Source: CAD feature listing. Evaluate the final solid. Frame: model axes, mm. A direction names the side the tool comes from. Coordinates: 2 decimals unless noted, no trailing zeros. Loops run counter-clockwise (first coordinate to the right, second up) from the corner with the lowest first, then second, coordinate; pieces in that order, holes last.
Item 1: Section query D-D, the plane x = 15. Return the cut outline in (y, z) (3 decimals).
Item 2: Section query B-B, the plane y = 2.5. Return the cut outline in (x, z) (3 decimals), then the cut area to 3 significant figures.
Item 3: Pull-direction query (Z, two-part tool) for faces 6 (the cylindrical face through (-8.926, -0.986, -41.626)), 7 (the flat face through (10.25, 7, -13)), 8 (the flat face through (0, -2, -53)); classes: +Z half, -Z half, draft (parallel to the pull), parting line (faces both ways), or undercut.
Item 4: Pin query (flat end, axial travel): pin 1 Ø5.5 at (x, z) = (-25.5, 24) entering from +Y; pin 2 Ø1 at (x, y) = (13.5, 9) entering from +Z; pin 3 Ø4 at (x, y) = (-1, 10) entering from -Z. Return the tip coordinate at first contact, or that it passes through.
Item 5: Reachability of faces 1 (the flat face through (-24.509, -1.479, -7.868)), 2 (the cylindrical face through (26.325, -2.535, -44.286)), 3 (the flat face through (-31, -2, -13)), 4 (the flat face through (20.4, 8, -11)), 5 (the flat face through (-14, 4.5, -13)) from +Z, -Z, +X, -X, +Y, -Y: full face, straight path, thin tool, end or side. Return the list, or none.
Item 6: Section query A-A, the plane z = -16. Return the cut outline in (x, y), then the cut area to 3 significant figures.
Item 7: Line query: probe 1 along X at (y, z) = (-3, -21.5); probe 2 along X at (y, z) = (-0.9, 24) (3 decimals); probe 3 along Z at (x, y) = (-21, -1.2). Output: solid intervals per line, ascending.
Item 8: Section query C-C, the plane z = 14. Return the cut outline in (x, y).
```python
from build123d import *

# Parameters (mm, degrees)
F1_W           = 31
F1_H           = 82
F2_DEPTH       = 5
F3_D           = 4.5
F3_CBORE_D     = 6.75
F3_CBORE_DEPTH = 2
F4_DEPTH       = 5
F5_DEPTH       = 2
F6_START       = 0.4
F0_R           = 1.35
F6_DEPTH       = 4.601
F7_D           = 3
F8_R           = 1.5
F9_DEPTH       = 3
F11_DEPTH      = 16.5
F15_D          = 4.25
F16_D          = 3
F18_R          = 2.125
F19_DEPTH      = 5.5
F20_W          = 3
F20_H          = 5
F21_DEPTH      = 3.75
F22_W          = 2.5
F22_H          = 5
F23_DEPTH      = 3.65
F24_R          = 1
F25_DEPTH      = 4
F25_DEPTH_BACK = 5.001
F26_R          = 0.3


# Not quite as in the source:
# - a pattern or mirror of a feature is missing from the dataset's text; its kind, count and spacing are read off the source's solid


with BuildPart() as f2:
    # F1 (on Front) → F2 (new body)
    with BuildSketch(Plane.XZ):
        with Locations((-15.5, -12)):
            Rectangle(F1_W, F1_H)
        with Locations((15.5, -12)):
            Rectangle(F1_W, F1_H)
    extrude(amount=F2_DEPTH)

    # F3 (through all)
    with Locations(Plane(origin=(0, 0, 0), x_dir=(1, 0, 0), z_dir=(0, 1, 0))):
        with Locations((24.75, -24), (6.75, -24), (-6.75, -24), (-24.75, -24), (-24.75, 0), (-6.75, 0), (6.75, 0), (24.75, 0)):
            CounterBoreHole(F3_D / 2, F3_CBORE_D / 2, F3_CBORE_DEPTH)

    # F0 (on Front) → F4 (cut, through all)
    with BuildSketch(Plane.XZ):
        with BuildLine():
            ThreePointArc((6.75, -23), (9, -25.25), (11.25, -23))
            Line((11.25, -23), (11.25, -21))
            ThreePointArc((11.25, -21), (9, -18.75), (6.75, -21))
            Line((6.75, -21), (6.75, -23))
        make_face()
        with BuildLine():
            Line((-6.75, -23), (-6.75, -21))
            ThreePointArc((-6.75, -21), (-9, -18.75), (-11.25, -21))
            Line((-11.25, -21), (-11.25, -23))
            ThreePointArc((-11.25, -23), (-9, -25.25), (-6.75, -23))
        make_face()
        with BuildLine():
            ThreePointArc((6.75, -47), (9, -49.25), (11.25, -47))
            Line((11.25, -47), (11.25, -45))
            ThreePointArc((11.25, -45), (9, -42.75), (6.75, -45))
            Line((6.75, -45), (6.75, -47))
        make_face()
        with BuildLine():
            Line((-6.75, -47), (-6.75, -45))
            ThreePointArc((-6.75, -45), (-9, -42.75), (-11.25, -45))
            Line((-11.25, -45), (-11.25, -47))
            ThreePointArc((-11.25, -47), (-9, -49.25), (-6.75, -47))
        make_face()
    extrude(amount=F4_DEPTH, mode=Mode.SUBTRACT)

    # F0 (on Front) → F5 (cut)
    with BuildSketch(Plane.XZ):
        with BuildLine():
            ThreePointArc((12.375, -21), (9, -17.625), (5.625, -21))
            Line((5.625, -21), (5.625, -23))
            ThreePointArc((5.625, -23), (9, -26.375), (12.375, -23))
            Line((12.375, -23), (12.375, -21))
        make_face()
        with BuildLine():
            Line((11.25, -21), (11.25, -23))
            ThreePointArc((11.25, -23), (9, -25.25), (6.75, -23))
            Line((6.75, -23), (6.75, -21))
            ThreePointArc((6.75, -21), (9, -18.75), (11.25, -21))
        make_face(mode=Mode.SUBTRACT)
        with BuildLine():
            Line((-5.625, -23), (-5.625, -21))
            ThreePointArc((-5.625, -21), (-9, -17.625), (-12.375, -21))
            Line((-12.375, -21), (-12.375, -23))
            ThreePointArc((-12.375, -23), (-9, -26.375), (-5.625, -23))
        make_face()
        with BuildLine():
            ThreePointArc((-11.25, -21), (-9, -18.75), (-6.75, -21))
            Line((-6.75, -21), (-6.75, -23))
            ThreePointArc((-6.75, -23), (-9, -25.25), (-11.25, -23))
            Line((-11.25, -23), (-11.25, -21))
        make_face(mode=Mode.SUBTRACT)
        with BuildLine():
            Line((-5.625, -47), (-5.625, -45))
            ThreePointArc((-5.625, -45), (-9, -41.625), (-12.375, -45))
            Line((-12.375, -45), (-12.375, -47))
            ThreePointArc((-12.375, -47), (-9, -50.375), (-5.625, -47))
        make_face()
        with BuildLine():
            ThreePointArc((-11.25, -45), (-9, -42.75), (-6.75, -45))
            Line((-6.75, -45), (-6.75, -47))
            ThreePointArc((-6.75, -47), (-9, -49.25), (-11.25, -47))
            Line((-11.25, -47), (-11.25, -45))
        make_face(mode=Mode.SUBTRACT)
        with BuildLine():
            ThreePointArc((12.375, -45), (9, -41.625), (5.625, -45))
            Line((5.625, -45), (5.625, -47))
            ThreePointArc((5.625, -47), (9, -50.375), (12.375, -47))
            Line((12.375, -47), (12.375, -45))
        make_face()
        with BuildLine():
            Line((11.25, -45), (11.25, -47))
            ThreePointArc((11.25, -47), (9, -49.25), (6.75, -47))
            Line((6.75, -47), (6.75, -45))
            ThreePointArc((6.75, -45), (9, -42.75), (11.25, -45))
        make_face(mode=Mode.SUBTRACT)
    extrude(amount=F5_DEPTH, mode=Mode.SUBTRACT)

    # F0 (on Front) → F6 (cut)
    with BuildSketch(Plane.XZ.offset(F6_START)):
        with Locations((-19, -21.5)):
            Circle(F0_R)
        with Locations((19, -21.5)):
            Circle(F0_R)
    extrude(amount=F6_DEPTH, mode=Mode.SUBTRACT)

    # F7 (through all)
    with Locations(Plane(origin=(0, 0, 0), x_dir=(1, 0, 0), z_dir=(0, 1, 0))):
        with Locations((26, 10.5), (-26, 10.5)):
            Hole(F7_D / 2)

    # F8 (on face) → F9 (cut)
    with BuildSketch(Plane(origin=(0, 0, 0), x_dir=(-1, 0, 0), z_dir=(0, 1, 0))):
        Polygon((29.025, -12.2464845643), (29.025, -8.7535154357), (26, -7.0070308714), (22.975, -8.7535154357), (22.975, -12.2464845643), (26, -13.9929691286), align=None)
        with Locations((26, -10.5)):
            Circle(F8_R, mode=Mode.SUBTRACT)
        Polygon((-22.975, -12.2464845643), (-22.975, -8.7535154357), (-26, -7.0070308714), (-29.025, -8.7535154357), (-29.025, -12.2464845643), (-26, -13.9929691286), align=None)
        with Locations((-26, -10.5)):
            Circle(F8_R, mode=Mode.SUBTRACT)
    extrude(amount=-F9_DEPTH, mode=Mode.SUBTRACT)

    # F10 (on face) → F11 (join)
    with BuildSketch(Plane(origin=(0, 0, 0), x_dir=(-1, 0, 0), z_dir=(0, 1, 0))):
        Polygon((-7.9, -5), (-20.4, -5), (-20.4, -17.25), (-7.9, -17.25), (-7.9, -14.7), (-5.9, -14.7), (-5.9, -8.7), (-7.9, -8.7), align=None)
        Polygon((0.1, -5), (-7.9, -5), (-7.9, -8.7), (-5.9, -8.7), (-5.9, -14.7), (-7.9, -14.7), (-7.9, -17.25), (0.1, -17.25), (20.6, -17.25), (20.6, -5), (1.3771316735, -5), align=None)
    extrude(amount=F11_DEPTH)

    # F12 (on face) → F13 (revolve, cut)
    with BuildSketch(Plane(origin=(0, 16.5, 0), x_dir=(-1, 0, 0), z_dir=(0, 1, 0))):
        Polygon((0.1, -5), (-7.9, -5), (-7.9, -8.7), (-5.9, -8.7), (-5.9, -14.7), (-7.9, -14.7), (-7.9, -17.25), (0.1, -17.25), align=None)
    revolve(axis=Axis((-0.1, 16.5, -11.8110565236), (0, 0, -1)), mode=Mode.SUBTRACT)

    # F15 (through all)
    with Locations(Plane(origin=(0, 16.5, 0), x_dir=(-1, 0, 0), z_dir=(0, 1, 0))):
        with Locations((-14, -11), (14, -10.5)):
            Hole(F15_D / 2)

    # F16 (through all)
    with Locations(Plane(origin=(0, 0, 0), x_dir=(1, 0, 0), z_dir=(0, 1, 0))):
        with Locations((26, 24.75), (21, 35.25), (26, 45.75), (-21, 35.25), (-26, 24.75), (-26, 45.75)):
            Hole(F16_D / 2)

    # F18 (on offset) → F19 (cut)
    with BuildSketch(Plane(origin=(0, 10, 0), x_dir=(-1, 0, 0), z_dir=(0, 1, 0))):
        Polygon((10.25, -12.6650635095), (10.25, -17.25), (17.75, -17.25), (17.75, -12.6650635095), (17.75, -8.3349364905), (14, -6.1698729811), (10.25, -8.3349364905), align=None)
        with Locations((14, -10.5)):
            Circle(F18_R, mode=Mode.SUBTRACT)
        Polygon((-10.25, -13.1650635095), (-10.25, -8.8349364905), (-14, -6.6698729811), (-17.75, -8.8349364905), (-17.75, -13.1650635095), (-17.75, -17.25), (-10.25, -17.25), align=None)
        with Locations((-14, -11)):
            Circle(F18_R, mode=Mode.SUBTRACT)
    extrude(amount=-F19_DEPTH, mode=Mode.SUBTRACT)

    # F20 (on face) → F21 (cut)
    with BuildSketch(Plane(origin=(0, 0, 0), x_dir=(-1, 0, 0), z_dir=(0, 1, 0))):
        with Locations((-25.85, 14.4774101714)):
            Rectangle(F20_W, F20_H)
        with Locations((25.85, 14.4774101714)):
            Rectangle(F20_W, F20_H)
    extrude(amount=-F21_DEPTH, mode=Mode.SUBTRACT)

    # F22 (on face) → F23 (cut, through all)
    with BuildSketch(Plane.YZ.offset(31)):
        with Locations((-2.5, 14.4774101714)):
            Rectangle(F22_W, F22_H)
    f23 = extrude(amount=-F23_DEPTH, mode=Mode.SUBTRACT)

    # F23_copies: F23 across plane
    add(f23.mirror(Plane(origin=(0, 0, 0), x_dir=(0, 0, -1), z_dir=(-1, 0, 0))), mode=Mode.SUBTRACT)

    # F24
    f24_edges = [f2.edges().sort_by_distance(p)[0] for p in [
        (24.35, -3.75, 14.47741),
        (27.35, -1.25, 14.47741),
        (-24.35, -3.75, 14.47741),
        (-27.35, -1.25, 14.47741),
    ]]
    fillet(f24_edges, radius=F24_R)

    # F0 (on Front) → F25 (cut, two sides)
    with BuildSketch(Plane.XZ) as f25_sk:
        with Locations((-19, -10.5)):
            Circle(F0_R)
        with Locations((19, -10.5)):
            Circle(F0_R)
    extrude(amount=-F25_DEPTH, mode=Mode.SUBTRACT)
    extrude(f25_sk.sketch, amount=F25_DEPTH_BACK, mode=Mode.SUBTRACT)

    # F26
    f26_edges = [f2.edges().sort_by_distance(p)[0] for p in [
        (-31, -2.5, 29),
        (31, -2.5, 29),
        (31, -2.5, -53),
        (-31, -2.5, -53),
        (-0.1, 10.5, -8.7),
        (-0.1, 10.5, -14.7),
    ]]
    fillet(f26_edges, radius=F26_R)


solid = f2.part
```
Verdict:
1. outline: (-5, -53) - (0, -53) - (0, -17.25) - (4.5, -17.25) - (4.5, -12.875) - (-5, -12.875) - close; (-5, -9.125) - (4.5, -9.125) - (4.5, -7.247) - (10, -7.247) - (10, -9.125) - (16.5, -9.125) - (16.5, -5) - (0, -5) - (0, 29) - (-5, 29) - close; (10, -17.25) - (16.5, -17.25) - (16.5, -12.875) - (10, -12.875) - close
2. outline: (-20.6, -17.25) - (20.4, -17.25) - (20.4, -5) - (-20.6, -5) - close; hole circle Ø2.7 at (-19, -10.5); hole circle Ø4.25 at (-14, -10.5); hole circle Ø4.25 at (14, -11); hole circle Ø2.7 at (19, -10.5)
2. area: 462 mm2
3. face 6: undercut
3. face 7: draft
3. face 8: -Z half
4. pin 1: stops at y = 0
4. pin 2: stops at z = -5
4. pin 3: stops at z = -17.25
5. face 1: +Y
5. face 2: +Y, -Y
5. face 3: +Z, -Z, -X, +Y, -Y
5. face 4: +Z, -Z, +X, +Y
5. face 5: -Z
6. outline: (-31, -5) - (31, -5) - (31, 0) - (20.4, 0) - (20.4, 16.5) - (7.9, 16.5) arc R8 cw to (-8.1, 16.5) - (-20.6, 16.5) - (-20.6, 0) - (-31, 0) - close; hole (-17.75, 4.5) - (-10.25, 4.5) - (-10.25, 10) - (-17.75, 10) - close; hole (10.25, 4.5) - (17.75, 4.5) - (17.75, 10) - (10.25, 10) - close
6. area: 803 mm2
7. probe 1: x = -31 to -20.35, -17.65 to -11.25, -6.75 to 6.75, 11.25 to 17.65, 20.35 to 31
7. probe 2: x = -31 to -28.125, -21.375 to -10.125, -3.375 to 3.375, 10.125 to 21.375, 28.125 to 31
7. probe 3: z = -53 to -36.75, -33.75 to 29
8. outline: (-31, -5) - (31, -5) - (31, -3.75) - (25.35, -3.75) arc R1 cw to (24.35, -2.75) - (24.35, 0) - (-24.35, 0) - (-24.35, -2.75) arc R1 cw to (-25.35, -3.75) - (-31, -3.75) - close; (-31, -1.25) - (-28.35, -1.25) arc R1 ccw to (-27.35, -0.25) - (-27.35, 0) - (-31, 0) - close; (27.35, -0.25) arc R1 ccw to (28.35, -1.25) - (31, -1.25) - (31, 0) - (27.35, 0) - close
